```python
from build123d import *

# Parameters (mm, degrees)
CROQUIS1_R              = 1.628014373
SALIENTE_EXTRUIR1_DEPTH = 4
SALIENTE_EXTRUIR2_DEPTH = 9
CROQUIS10_R             = 1
CORTAR_EXTRUIR3_DEPTH   = 4
SALIENTE_EXTRUIR3_DEPTH = 20
SALIENTE_EXTRUIR4_DEPTH = 20
CROQUIS17_R             = 1.5
CORTAR_EXTRUIR6_DEPTH   = 4
CROQUIS19_W             = 20
CROQUIS19_H             = 4
CORTAR_EXTRUIR7_DEPTH   = 2


with BuildPart() as part:
    # Croquis1 → Saliente-Extruir1 (new body)
    with BuildSketch(Plane.XY):
        with BuildLine():
            Line((-79.034482165, 42.285614206), (-79.034482165, 34.285614206))
            Line((-79.034482165, 34.285614206), (-85.534482165, 34.285614206))
            Line((-85.534482165, 34.285614206), (-85.534482165, 43.91362858))
            ThreePointArc((-85.534482165, 43.91362858), (-89.034482165, 47.41362858), (-92.534482165, 43.91362858))
            Line((-92.534482165, 43.91362858), (-92.534482165, 34.285614206))
            Line((-92.534482165, 34.285614206), (-99.034482165, 34.285614206))
            Line((-99.034482165, 34.285614206), (-99.034482165, 42.285614206))
            Line((-99.034482165, 42.285614206), (-99.034482165, 54.285614206))
            Line((-99.034482165, 54.285614206), (-79.034482165, 54.285614206))
            Line((-79.034482165, 54.285614206), (-79.034482165, 42.285614206))
        make_face()
        with Locations((-96.034482165, 38.285614206)):
            Circle(CROQUIS1_R, mode=Mode.SUBTRACT)
        with Locations((-82.034482165, 38.285614206)):
            Circle(CROQUIS1_R, mode=Mode.SUBTRACT)
    extrude(amount=SALIENTE_EXTRUIR1_DEPTH)

    # Croquis2 → Saliente-Extruir2 (add)
    with BuildSketch(Plane(origin=(0, 0, 0), x_dir=(-1, 0, 0), z_dir=(0, 0, -1))):
        with BuildLine():
            Line((79.034482165, 41.131975098), (83.718242525, 41.131975098))
            ThreePointArc((83.718242525, 41.131975098), (89.034482165, 49.91362858), (94.350721805, 41.131975098))
            Line((94.350721805, 41.131975098), (99.034482165, 41.131975098))
            Line((99.034482165, 41.131975098), (99.034482165, 54.285614206))
            Line((99.034482165, 54.285614206), (79.034482165, 54.285614206))
            Line((79.034482165, 54.285614206), (79.034482165, 41.131975098))
        make_face()
    extrude(amount=SALIENTE_EXTRUIR2_DEPTH)

    # Croquis10 → Cortar-Extruir3 (cut)
    with BuildSketch(Plane(origin=(0, 0, -9), x_dir=(-1, 0, 0), z_dir=(0, 0, -1))):
        with Locations((96.534482165, 51.785614206)):
            Circle(CROQUIS10_R)
        with Locations((81.034482165, 43.131975098)):
            Circle(CROQUIS10_R)
    extrude(amount=-CORTAR_EXTRUIR3_DEPTH, mode=Mode.SUBTRACT)

    # Croquis11 → Saliente-Extruir3 (add)
    with BuildSketch(Plane.ZY.offset(99.034482165)):
        Polygon((-9, 54.285614206), (-9, 61.791167706), (4, 54.285614206), align=None)
    extrude(amount=-SALIENTE_EXTRUIR3_DEPTH)

    # Croquis16 → Saliente-Extruir4 (add)
    with BuildSketch(Plane.ZY.offset(99.034482165)):
        Polygon((-9, 61.791167706), (-21.990381057, 69.291167706), (-22.990381057, 67.559116898), (-9, 59.481766629), align=None)
    extrude(amount=-SALIENTE_EXTRUIR4_DEPTH)

    # Croquis17 → Cortar-Extruir6 (cut)
    with BuildSketch(Plane(origin=(0, 42.446261462, 24.506360481), x_dir=(1, 0, 0), z_dir=(0, 0.8660254037844418, 0.49999999999999484))):
        with Locations(Location((-84.034482165, 33.684258988, 0), (0, 0, 270))):
            Circle(CROQUIS17_R)
        with Locations(Location((-94.034482165, 33.684258988, 0), (0, 0, 270))):
            Circle(CROQUIS17_R)
        with Locations(Location((-94.034482165, 43.684258988, 0), (0, 0, 270))):
            Circle(CROQUIS17_R)
        with Locations(Location((-84.034482165, 43.684258988, 0), (0, 0, 270))):
            Circle(CROQUIS17_R)
    extrude(amount=-CORTAR_EXTRUIR6_DEPTH, mode=Mode.SUBTRACT)

    # Croquis19 → Cortar-Extruir7 (cut)
    with BuildSketch(Plane(origin=(0, 42.446261462, 24.506360481), x_dir=(1, 0, 0), z_dir=(0, 0.8660254037844418, 0.49999999999999484))):
        with Locations((-89.034482165, 51.689812487)):
            Rectangle(CROQUIS19_W, CROQUIS19_H)
    extrude(amount=-CORTAR_EXTRUIR7_DEPTH, mode=Mode.SUBTRACT)


solid = part.part
```
Model file for the job. Use its own axes, mm. A direction names the side the tool comes from. Round coordinates to 2 decimals unless told otherwise and drop trailing zeros. Order: outer loops, then holes, each group sorted by start corner. A loop starts at its lowest first (then second) coordinate and runs counter-clockwise, first axis right, second up. Notation, with made-up numbers: M 45.25,74 L 56.25,74 A27 cw 56.25,94 Z; hole C 0.5,-20 d5. An arc over 180 degrees is marked long. Use CSV: the item, a comma, the result in double quotes.
Item 1: Which spindle directions (+Z, -Z, +X, -X, +Y, -Y) get a long thin tool onto all of the face, cutting with end or side? Do faces 1 (the face through (-85.534, 39, 2)), 2 (the face through (-89, 52, -9)), 3 (the face through (-97, 52, -5)). Say none if no direction does.
Worked answers:
face 1,"+Z, -Z, -Y"
face 2,"-Z, +X, -X, -Y"
face 3,"-Z"
Item 2: Pull direction Z, two halves, no side cores. Call faces 4 (the face through (-85.5, 57.74, -5.93)), 5 (the face through (-97, 41.132, -4)), 6 (the face through (-89.174, 62.563, -14.337)): released by +Z, released by -Z, zero draft, split by the parting line, or undercut.
Worked answers:
face 4,"undercut"
face 5,"zero draft"
face 6,"released by -Z"
Item 3: Saw through at A-A (y = 39.5). List the corners of the cut face in (x, z).
Worked answers:
outline,"M -99.03,0 L -97.12,0 L -97.12,4 L -99.03,4 Z; M -94.95,0 L -92.53,0 L -92.53,4 L -94.95,4 Z; M -85.53,0 L -83.12,0 L -83.12,4 L -85.53,4 Z; M -80.95,0 L -79.03,0 L -79.03,4 L -80.95,4 Z"
Item 4: Saw through at D-D (y = 48.5). List the corners of the cut face in (x, z).
Worked answers:
outline,"M -99.03,-9 L -92.9,-9 L -92.9,0 L -85.17,0 L -85.17,-9 L -79.03,-9 L -79.03,4 L -99.03,4 Z"
Item 5: Pin check, flat tips, straight feed: pin 1 (5 mm diameter, centred on x = -96.03, y = 38.29, fed in from -Z); pin 2 (10 mm diameter, centred on x = -83, z = -8, fed in from +Y); pin 3 (3.5 mm diameter, centred on x = -96.5, z = -4, fed in from -Y); pin 4 (1 mm diameter, centred on y = 42, z = -10, fed in from -X). Stop position of each tip, or through.
Worked answers:
pin 1,"z = 0"
pin 2,"y = 64.09"
pin 3,"y = 41.13"
pin 4,"through"
Item 6: Probe probe 1 along Z at (x, y) = (-97.5, 43); probe 2 along Y at (x, z) = (-83, 0.25); probe 3 along X at (y, z) = (46.5, 3.25). List the from-to ranges inside material, lowest first.
Worked answers:
probe 1,"-9 to 4"
probe 2,"34.29 to 36.97, 39.6 to 56.45"
probe 3,"-99.03 to -91.39, -86.68 to -79.03"
Item 7: Saw through at C-C (y = 44.5). List the corners of the cut face in (x, z), plus the area to 3 significant figures.
Worked answers:
outline,"M -99.03,-9 L -95.01,-9 L -95.01,0 L -92.49,0 L -92.49,4 L -99.03,4 Z; M -85.58,0 L -83.06,0 L -83.06,-9 L -79.03,-9 L -79.03,4 L -85.58,4 Z"
area,"125 mm²"
Item 8: Saw through at B-B (x = -86). List the corners of the cut face in (y, z), plus the area to 3 significant figures.
Worked answers:
outline,"M 45.66,0 L 49.09,0 L 49.09,-9 L 59.48,-9 L 65.56,-19.53 L 67.29,-18.53 L 54.29,4 L 45.66,4 Z"
area,"153 mm²"
